Geometry check sheet. Reference: the model listing, model coordinates, mm. A direction names the side the tool comes from. Coordinates: 2 decimals unless noted, no trailing zeros. Loops run counter-clockwise (first coordinate to the right, second up) from the corner with the lowest first, then second, coordinate; pieces in that order, holes last. Notation, with made-up numbers: (33, -31) - (68, -31) arc R16 ccw to (68, -6) - close; hole circle Ø11 at (20, 88.25). An arc over 180 degrees is marked (long way). Write each question's results on one line, items separated by ' | '. Start each with the question number.
(1) Go/stop test with flat-tipped pins: pin 1 Ø8 at (x, y) = (2.5, 16) entering from -Z; pin 2 Ø6.5 at (y, z) = (28, 20.5) entering from +X; pin 3 Ø10 at (x, y) = (-9.5, -6.5) entering from +Z; pin 4 Ø2 at (x, z) = (8, 11.5) entering from +Y. Record where each tip stops, or that it passes through.
(2) Access from +Z, -Z, +X, -X, +Y, -Y to the whole of each face (thin tool, end or side, straight path). Record for faces 1 (the face through (-5, 19, 0)), 2 (the face through (-6.35, 26, 25)), 3 (the face through (6.35, 27, 25)), 4 (the face through (-3.175, 25, 25)), 5 (the face through (5, 31.75, 25)).
(3) Mould release check, pull along Y, two halves, no side actions. Record for faces 6 (the face through (3.175, 25, 25)), 7 (the face through (0.887, -22.207, 25.044)), 8 (the face through (-0.793, -19.033, 25.044)): pulls with the +Y half, pulls with the -Y half, needs draft (parallel to the pull), parting line crosses it, or undercut.
(4) Material ranges on probe 1 along X at (y, z) = (0.5, 24); probe 2 along Y at (x, z) = (0, 38) (3 decimals); probe 3 along X at (y, z) = (-15.5, 16.5), recorded low to high.
(5) Sectioned sample at D-D (x = 0). Enter the section's corners in (y, z) (3 decimals), plus the area to 3 significant figures.
(6) Sectioned sample at A-A (y = 0). Enter the section's corners in (x, z) (3 decimals).
(7) Sectioned sample at C-C (x = 17.5). Enter the section's corners in (y, z), plus the area to 3 significant figures.
(8) Sectioned sample at B-B (z = 26). Enter the section's corners in (x, y) (3 decimals), plus the area to 3 significant figures.
from build123d import *

# Parameters (mm, degrees)
BOSS_EXTRUDE1_DEPTH = 50.8


with BuildPart() as part:
    # Sketch2 → Boss-Extrude1 (new body)
    with BuildSketch(Plane.XY):
        with BuildLine():
            Line((3.175, 22.86), (3.175, 31.75))
            Line((3.175, 31.75), (6.35, 31.75))
            Line((6.35, 31.75), (6.35, 21.298547486))
            ThreePointArc((6.35, 21.298547486), (0, -22.225), (-6.35, 21.298547486))
            Line((-6.35, 21.298547486), (-6.35, 31.75))
            Line((-6.35, 31.75), (-3.175, 31.75))
            Line((-3.175, 31.75), (-3.175, 22.86))
            Line((-3.175, 22.86), (-3.175, 18.783553311))
            ThreePointArc((-3.175, 18.783553311), (0, -19.05), (3.175, 18.783553311))
            Line((3.175, 18.783553311), (3.175, 22.86))
        make_face()
    extrude(amount=BOSS_EXTRUDE1_DEPTH)


solid = part.part
Outcome:
1) pin 1: stops at z = 0 | pin 2: stops at x = 6.35 | pin 3: passes through | pin 4: stops at y = 21.09
2) face 1: -Z, +X, -X, +Y, -Y | face 2: +Z, -Z, -X, +Y | face 3: +Z, -Z, +X, +Y | face 4: +Z, -Z, +Y | face 5: +Z, -Z, +X, -X, +Y
3) face 6: needs draft | face 7: parting line crosses it | face 8: undercut
4) probe 1: x = -22.22 to -19.04, 19.04 to 22.22 | probe 2: y = -22.225 to -19.05 | probe 3: x = -15.93 to -11.07, 11.07 to 15.93
5) outline: (-22.225, 0) - (-19.05, 0) - (-19.05, 50.8) - (-22.225, 50.8) - close | area: 161 mm2
6) outline: (-22.225, 0) - (-19.05, 0) - (-19.05, 50.8) - (-22.225, 50.8) - close; (19.05, 0) - (22.225, 0) - (22.225, 50.8) - (19.05, 50.8) - close
7) outline: (-13.7, 0) - (-7.53, 0) - (-7.53, 50.8) - (-13.7, 50.8) - close; (7.53, 0) - (13.7, 0) - (13.7, 50.8) - (7.53, 50.8) - close | area: 627 mm2
8) outline: (-6.35, 21.299) arc R22.225 ccw (long way) to (6.35, 21.299) - (6.35, 31.75) - (3.175, 31.75) - (3.175, 18.784) arc R19.05 cw (long way) to (-3.175, 18.784) - (-3.175, 31.75) - (-6.35, 31.75) - close | area: 455 mm2
